Source: CAD feature listing. Evaluate the final solid. Frame: model axes, mm. A direction names the side the tool comes from. Coordinates: 2 decimals unless noted, no trailing zeros. Order: outer loops, then holes, each group sorted by start corner. A loop starts at its lowest first (then second) coordinate and runs counter-clockwise, first axis right, second up. Notation, with made-up numbers: (59.25, -21.75) -> (104.25, -21.75) arc R21 cw to (104.25, 15.25) -> close; hole circle Ø2 at (-38, 19.5). An arc over 180 degrees is marked (long way). Write item = value, one per line. Start each with the question number.
Item 1: Section query C-C (x = 27). Output: boundary loops of the cut face in (y, z).
Item 2: Section query D-D (z = 0.65). Output: boundary loops of the cut face in (x, y).
Item 3: Mould query, pull axis Y, two halves, no side actions, for faces 4 (the flat face through (2.89, -4.99, 2.54)), 5 (the flat face through (0, -10, 2)), 6 (the flat face through (2.864, 5.015, 2.535)), 7 (the flat face through (-25, -12, 1.5)). Classes: released by +Y, released by -Y, zero draft, split by the parting line, or undercut.
Item 4: Set-up query: faces 1 (the flat face through (17.136, -5.015, 2.535)), 2 (the flat face through (-25, -12, 3.5)), 3 (the flat face through (25, 12, 1.5)). Return all of +Z, -Z, +X, -X, +Y, -Y with unobstructed straight access to the full face (end or side cutting, diameter ignored); none if empty.
Item 5: Ray query, line 1 along X through (y, z) = (-6.25, 4.5); line 2 along X through (y, z) = (-4.25, 0.5); line 3 along Y through (x, z) = (-21, 4.5). Return the intervals inside material, ascending. Write a range as [from, to].
Item 6: Contact query for flat-ended pins moving along their axis: pin 1 (4 mm diameter, centred on x = -25.5, y = 13.5, fed in from -Z); pin 2 (2 mm diameter, centred on x = -15, z = 3, fed in from +Y); pin 3 (5.5 mm diameter, centred on x = -26, y = -13.5, fed in from +Z). Output: stop coordinate, or through.
Item 7: Section query A-A (x = 10). Output: boundary loops of the cut face in (y, z).
```python
from build123d import *

# Parameters (mm, degrees)
F0_W     = 70
F0_H     = 20
F1_DEPTH = 5
F2_W     = 10
F2_H     = 2
F3_DEPTH = 5
F4_W     = 10
F4_H     = 2
F5_DEPTH = 5
F6_R     = 0.99999
F7_R     = 2.49999
F9_DEPTH = 5


# Not quite as in the source:
# - a fillet or chamfer is up to 0.001 mm smaller than in the source, because OpenCascade refuses the exact size


with BuildPart() as f1:
    # F0 (on Top) → F1 (new body)
    with BuildSketch(Plane.XY):
        Rectangle(F0_W, F0_H)
    extrude(amount=F1_DEPTH)

    # F2 (on face) → F3 (join)
    with BuildSketch(Plane.XZ.offset(10)):
        with Locations((-25, 2.5)):
            Rectangle(F2_W, F2_H)
        with Locations((25, 2.5)):
            Rectangle(F2_W, F2_H)
    extrude(amount=F3_DEPTH)

    # F4 (on face) → F5 (join)
    with BuildSketch(Plane(origin=(0, 10, 0), x_dir=(-1, 0, 0), z_dir=(0, 1, 0))):
        with Locations((-25, 2.5)):
            Rectangle(F4_W, F4_H)
        with Locations((25, 2.5)):
            Rectangle(F4_W, F4_H)
    extrude(amount=F5_DEPTH)

    # F6 (radius 1 in the source; OpenCascade refuses exactly that, so slightly less here)
    f6_edges = [f1.edges().sort_by_distance(p)[0] for p in [
        (30, 12.5, 3.5),
        (30, 12.5, 1.5),
        (20, 12.5, 3.5),
        (30, -12.5, 3.5),
        (30, -12.5, 1.5),
        (20, -12.5, 3.5),
        (-20, 12.5, 3.5),
        (-20, 12.5, 1.5),
        (-30, -12.5, 3.5),
        (-20, -12.5, 3.5),
        (-20, -12.5, 1.5),
        (-30, 12.5, 3.5),
        (20, 12.5, 1.5),
        (-30, 12.5, 1.5),
        (-30, -12.5, 1.5),
        (20, -12.5, 1.5),
    ]]
    fillet(f6_edges, radius=F6_R)

    # F7 (radius 2.5 in the source; OpenCascade refuses exactly that, so slightly less here)
    f7_edges = [f1.edges().sort_by_distance(p)[0] for p in [
        (35, 0, 5),
        (35, 0, 0),
    ]]
    fillet(f7_edges, radius=F7_R)

    # F8 (on face) → F9 (cut)
    with BuildSketch(Plane.XY.offset(5)):
        with BuildLine():
            Line((6.0606601718, -3.9393398282), (1.8180194847, -8.1819805153))
            ThreePointArc((1.8180194847, -8.1819805153), (2.8786796564, -8.6213203436), (3.9393398282, -8.1819805153))
            Line((3.9393398282, -8.1819805153), (6.0606601718, -6.0606601718))
            ThreePointArc((6.0606601718, -6.0606601718), (6.5, -5), (6.0606601718, -3.9393398282))
        make_face()
        with BuildLine():
            ThreePointArc((1.8180194847, -6.0606601718), (1.3786796564, -7.1213203436), (1.8180194847, -8.1819805153))
            Line((1.8180194847, -8.1819805153), (6.0606601718, -3.9393398282))
            ThreePointArc((6.0606601718, -3.9393398282), (5, -3.5), (3.9393398282, -3.9393398282))
            Line((3.9393398282, -3.9393398282), (1.8180194847, -6.0606601718))
        make_face()
        with BuildLine():
            ThreePointArc((7.1715728753, 2.8284271247), (6.30448187, 1.5307337295), (6, 0))
            Line((6, 0), (10, 0))
            Line((10, 0), (7.1715728753, 2.8284271247))
        make_face()
        with BuildLine():
            Line((10, 0), (6, 0))
            ThreePointArc((6, 0), (6.30448187, -1.5307337295), (7.1715728753, -2.8284271247))
            Line((7.1715728753, -2.8284271247), (10, 0))
        make_face()
        with BuildLine():
            Line((12.8284271247, -2.8284271247), (10, 0))
            Line((10, 0), (7.1715728753, -2.8284271247))
            ThreePointArc((7.1715728753, -2.8284271247), (10, -4), (12.8284271247, -2.8284271247))
        make_face()
        with BuildLine():
            Line((13.9393398282, -3.9393398282), (18.1819805153, -8.1819805153))
            ThreePointArc((18.1819805153, -8.1819805153), (18.6213203436, -7.1213203436), (18.1819805153, -6.0606601718))
            Line((18.1819805153, -6.0606601718), (16.0606601718, -3.9393398282))
            ThreePointArc((16.0606601718, -3.9393398282), (15, -3.5), (13.9393398282, -3.9393398282))
        make_face()
        with BuildLine():
            ThreePointArc((16.0606601718, -8.1819805153), (17.1213203436, -8.6213203436), (18.1819805153, -8.1819805153))
            Line((18.1819805153, -8.1819805153), (13.9393398282, -3.9393398282))
            ThreePointArc((13.9393398282, -3.9393398282), (13.5, -5), (13.9393398282, -6.0606601718))
            Line((13.9393398282, -6.0606601718), (16.0606601718, -8.1819805153))
        make_face()
        with BuildLine():
            ThreePointArc((18.1819805153, 6.0606601718), (18.6213203436, 7.1213203436), (18.1819805153, 8.1819805153))
            ThreePointArc((18.1819805153, 8.1819805153), (17.1213203436, 8.6213203436), (16.0606601718, 8.1819805153))
            Line((16.0606601718, 8.1819805153), (13.9393398282, 6.0606601718))
            ThreePointArc((13.9393398282, 6.0606601718), (13.5, 5), (13.9393398282, 3.9393398282))
            ThreePointArc((13.9393398282, 3.9393398282), (15, 3.5), (16.0606601718, 3.9393398282))
            Line((16.0606601718, 3.9393398282), (18.1819805153, 6.0606601718))
        make_face()
        with BuildLine():
            ThreePointArc((3.9393398282, 8.1819805153), (2.8786796564, 8.6213203436), (1.8180194847, 8.1819805153))
            ThreePointArc((1.8180194847, 8.1819805153), (1.3786796564, 7.1213203436), (1.8180194847, 6.0606601718))
            Line((1.8180194847, 6.0606601718), (3.9393398282, 3.9393398282))
            ThreePointArc((3.9393398282, 3.9393398282), (5, 3.5), (6.0606601718, 3.9393398282))
            ThreePointArc((6.0606601718, 3.9393398282), (6.5, 5), (6.0606601718, 6.0606601718))
            Line((6.0606601718, 6.0606601718), (3.9393398282, 8.1819805153))
        make_face()
        with BuildLine():
            Line((7.1715728753, 2.8284271247), (10, 0))
            Line((10, 0), (12.8284271247, 2.8284271247))
            ThreePointArc((12.8284271247, 2.8284271247), (10, 4), (7.1715728753, 2.8284271247))
        make_face()
        with BuildLine():
            Line((12.8284271247, 2.8284271247), (10, 0))
            Line((10, 0), (14, 0))
            ThreePointArc((14, 0), (13.69551813, 1.5307337295), (12.8284271247, 2.8284271247))
        make_face()
        with BuildLine():
            Line((14, 0), (10, 0))
            Line((10, 0), (12.8284271247, -2.8284271247))
            ThreePointArc((12.8284271247, -2.8284271247), (13.69551813, -1.5307337295), (14, 0))
        make_face()
    extrude(amount=-F9_DEPTH, mode=Mode.SUBTRACT)


solid = f1.part
```
Computed:
q1.outline = (-15, 1.5) -> (-10, 1.5) -> (-10, 0) -> (10, 0) -> (10, 1.5) -> (15, 1.5) -> (15, 3.5) -> (10, 3.5) -> (10, 5) -> (-10, 5) -> (-10, 3.5) -> (-15, 3.5) -> close
q2.outline = (-35, -10) -> (34.18, -10) -> (34.18, 10) -> (-35, 10) -> close; hole (1.82, -6.06) arc R1.5 ccw to (3.94, -8.18) -> (6.06, -6.06) arc R1.5 ccw to (3.94, -3.94) -> close; hole (1.82, 6.06) -> (3.94, 3.94) arc R1.5 ccw to (6.06, 6.06) -> (3.94, 8.18) arc R1.5 ccw to start; hole circle Ø8 at (10, 0); hole (13.94, -6.06) -> (16.06, -8.18) arc R1.5 ccw to (18.18, -6.06) -> (16.06, -3.94) arc R1.5 ccw to start; hole (13.94, 6.06) arc R1.5 ccw to (16.06, 3.94) -> (18.18, 6.06) arc R1.5 ccw to (16.06, 8.18) -> close
q3.face_4 = undercut
q3.face_5 = released by -Y
q3.face_6 = undercut
q3.face_7 = zero draft
q4.face_1 = +Z, -Z
q4.face_2 = +Z, +X, -X, -Y
q4.face_3 = -Z, +X, -X, +Y
q5.line_1 = [-35, 1.66], [5.87, 14.13], [18.34, 34]
q5.line_2 = [-35, 3.63], [6.3, 13.7], [16.37, 34]
q5.line_3 = [-10, 10]
q6.pin_1 = 1.5
q6.pin_2 = 10
q6.pin_3 = 3.5
q7.outline = (-10, 0) -> (-4, 0) -> (-4, 5) -> (-10, 5) -> close; (4, 0) -> (10, 0) -> (10, 5) -> (4, 5) -> close
